The drawing under review shows one solid part. Ordinate dimensions are in mm from its lowest x, y, z. Give positions to 0.01 mm unless a question says otherwise; leave off trailing zeros. Write each loop counter-clockwise with the first axis right and the second up, starting at its lowest first coordinate (ties: lowest second). Pieces come first, ordered by that corner, then holes. Notation, with made-up numbers: M 14,-4 L 57,-4 A24 cw 57,12 Z; hole C 74.25,39 d8. An arc over 180 degrees is marked long. Use one line per item in the form item = value. Start each with the question number.
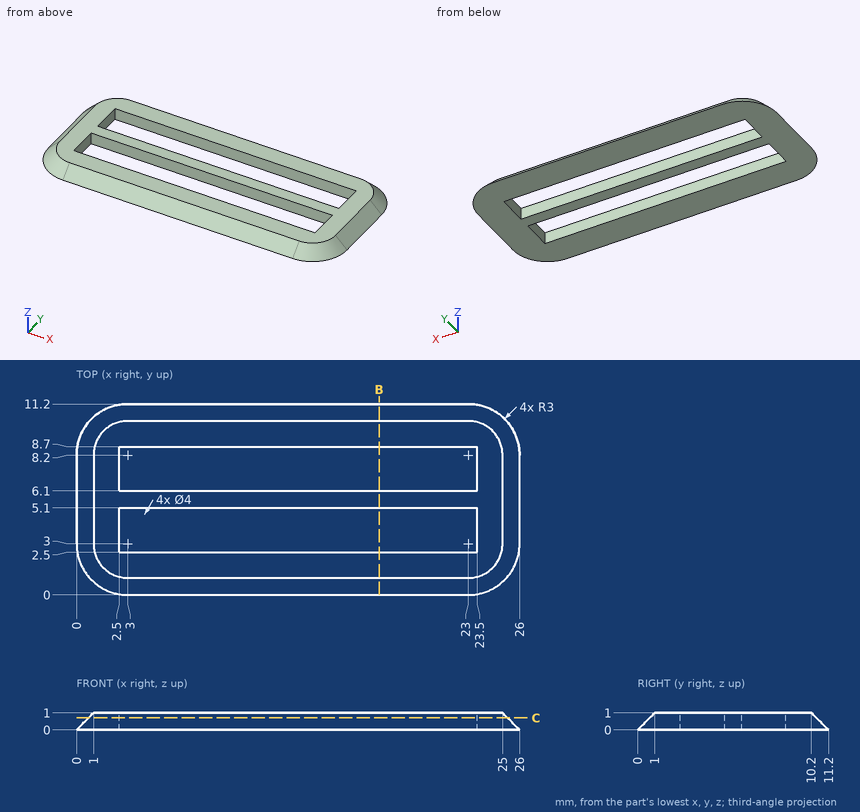
1. We need section B-B (x = 17.75). Give the number of separate pieces and of enclosed holes in the cut face, and give its area (3 significant figures).
2. We need section C-C (z = 0.7). State the section outline as (x, y) points, and give its area (3 significant figures).
3. To check wall thickness, follow L1, parallel to Y at x = 13.5, z = 0.15; L2, parallel to Y at x = 18.75, z = 0.7; L3, parallel to X at y = 6.75, z = 0.85. State the ranges of each line that lie inside material, in increasing order.
4. Clearance check with flat-ended pins moving along their axes: pin 1 Ø0.5 at (y, z) = (3.5, 0.5) entering from +X; pin 2 Ø6 at (x, y) = (22, 2.5) entering from -Z; pin 3 Ø0.5 at (x, z) = (16.5, 0.5) entering from +Y; pin 4 Ø0.5 at (x, z) = (9.5, 0.5) entering from -Y. State where each tip first meets the part, or that it passes through.
Answer block:
q1.separate_pieces = 3
q1.enclosed_holes = 0
q1.area = 5.00 mm^2
q2.outline = M 0.7,3 A2.3 ccw 3,0.7 L 23,0.7 A2.3 ccw 25.3,3 L 25.3,8.2 A2.3 ccw 23,10.5 L 3,10.5 A2.3 ccw 0.7,8.2 Z; hole M 2.5,2.5 L 23.5,2.5 L 23.5,5.1 L 2.5,5.1 Z; hole M 2.5,6.1 L 23.5,6.1 L 23.5,8.7 L 2.5,8.7 Z
q2.area = 127 mm^2
q3.L1 = 0.15 to 2.5, 5.1 to 6.1, 8.7 to 11.05
q3.L2 = 0.7 to 2.5, 5.1 to 6.1, 8.7 to 10.5
q3.L3 = 0.85 to 2.5, 23.5 to 25.15
q4.pin_1 = 25.75
q4.pin_2 = 0
q4.pin_3 = 10.95
q4.pin_4 = 0.25
